CAD build for the part. Positions are in the model's coordinates, mm. A direction names the side the tool comes from. Give positions to 0.01 mm unless a question says otherwise; leave off trailing zeros. Write each loop counter-clockwise with the first axis right and the second up, starting at its lowest first coordinate (ties: lowest second). Pieces come first, ordered by that corner, then holes. Notation, with made-up numbers: (26.5, 36) - (82.5, 36) arc R16 cw to (82.5, 50) - close; hole circle Ø10 at (4, -5.75). An arc over 180 degrees is marked (long way). Answer as a JSON object with one key per item and string values.
from build123d import *

# Parameters (mm, degrees)
F1_DEPTH = 37.5
F2_DEPTH = 20
F4_DEPTH = 70
F3_R     = 5
F5_DEPTH = 30
F6_R     = 20
F7_DEPTH = 100


with BuildPart() as f1:
    # F0 (on Front) → F1 (new body, symmetric)
    with BuildSketch(Plane.XZ):
        with BuildLine():
            ThreePointArc((10.173274, -20.068744), (19.172228, -11.776064), (22.5, 0))
            ThreePointArc((22.5, 0), (19.172228, 11.776064), (10.173274, 20.068744))
            ThreePointArc((10.173274, 20.068744), (-22.5, 0), (10.173274, -20.068744))
        make_face()
    extrude(amount=F1_DEPTH, both=True)

    # F0 (on Front) → F2 (join, symmetric)
    with BuildSketch(Plane.XZ):
        with BuildLine():
            ThreePointArc((10.173274, 20.068744), (19.172228, 11.776064), (22.5, 0))
            ThreePointArc((22.5, 0), (19.172228, -11.776064), (10.173274, -20.068744))
            Line((10.173274, -20.068744), (42.5, -20.285756))
            Line((42.5, -20.285756), (42.5, 0))
            Line((42.5, 0), (42.5, 20.285756))
            Line((42.5, 20.285756), (10.173274, 20.068744))
        make_face()
    extrude(amount=F2_DEPTH, both=True)

    # F3 (on face) → F4 (cut)
    with BuildSketch(Plane(origin=(-0.134258, 0, 19.999549), x_dir=(0.999977, 0, 0.006713), z_dir=(-0.006713, 0, 0.999977))):
        with BuildLine():
            ThreePointArc((40.021521, 5.68982), (41.950542, 3.130714), (42.635219, 0))
            Line((42.635219, 0), (42.635219, 20))
            Line((42.635219, 20), (23.358133, 20))
            Line((23.358133, 20), (40.021521, 5.68982))
        make_face()
        with BuildLine():
            Line((42.635219, -20), (42.635219, 0))
            ThreePointArc((42.635219, 0), (41.950542, -3.130714), (40.021521, -5.68982))
            Line((40.021521, -5.68982), (23.358133, -20))
            Line((23.358133, -20), (42.635219, -20))
        make_face()
    extrude(amount=-F4_DEPTH, mode=Mode.SUBTRACT)

    # F3 (on face) → F5 (cut)
    with BuildSketch(Plane(origin=(-0.134258, 0, 19.999549), x_dir=(0.999977, 0, 0.006713), z_dir=(-0.006713, 0, 0.999977))):
        with Locations((35.135219, 0)):
            Circle(F3_R)
    extrude(amount=-F5_DEPTH, mode=Mode.SUBTRACT)

    # F6 (on face) → F7 (cut)
    with BuildSketch(Plane.XZ.offset(37.5)):
        Circle(F6_R)
    extrude(amount=-F7_DEPTH, mode=Mode.SUBTRACT)


solid = f1.part
Item 1: Cut at C-C (z = 17). State how many separate pieces and enclosed holes the cut face has, and give its area (3 significant figures).
Entries:
{"separate pieces": "2", "enclosed holes": "1", "area": "1,340 mm2"}
Item 2: Probe line 1 (Z direction, x = 0, y = -22); line 2 (X direction, y = 0.5, z = 7.5); line 3 (X direction, y = 23.5, z = -3). List the from-to ranges inside material, lowest first. Write a range as from..to.
Entries:
{"line 1": "-22.5..-20, 20..22.5", "line 2": "-21.21..-18.54, 18.54..30.11, 40.06..42.5", "line 3": "-22.3..-19.77, 19.77..22.3"}
Item 3: Which spindle directions (+Z, -Z, +X, -X, +Y, -Y) get a long thin tool onto all of the face, cutting with end or side? Do faces 1 (the flat face through (23, -20, 2)), 2 (the cylindrical face through (41.6, 3.8, 0.3)), 3 (the flat face through (42.5, 0, -5)), 4 (the flat face through (23, 20, 2)), 5 (the flat face through (-20.1, -37.5, -1.6)). Say none if no direction does.
Entries:
{"face 1": "+X, -Y", "face 2": "+Z, +X, +Y", "face 3": "+Z, -Z, +X, +Y, -Y", "face 4": "+X, +Y", "face 5": "+Z, -Z, +X, -X, -Y"}
Item 4: Mould opens along X. For faces 6 (the cylindrical face through (41.64, -3.73, 0.28)), 7 (the flat face through (-20.1, 37.5, -1.6)), 8 (the cylindrical face through (-4.336, -0.525, -19.524)), 9 (the cylindrical face through (30.104, 0.22, 5.412)) say: +X half, -X half, draft (parallel to the pull), parting line (faces both ways), or undercut.
Entries:
{"face 6": "+X half", "face 7": "draft", "face 8": "undercut", "face 9": "undercut"}
Item 5: Cut at D-D (x = -16.5). Give the cut face in (y, z), and give its area (3 significant figures).
Entries:
{"outline": "(-37.5, -15.3) - (37.5, -15.3) - (37.5, -11.3) - (-37.5, -11.3) - close; (-37.5, 11.3) - (37.5, 11.3) - (37.5, 15.3) - (-37.5, 15.3) - close", "area": "599 mm2"}
Item 6: Flat gauge pins, fed straight in: P1, Ø1, axis at y = -22, z = 9.5, coming from the +X side; P2, Ø12, axis at x = 20.5, y = -28, coming from the -Z side; P3, Ø6, axis at x = 25, z = 9, coming from the -Y side. Where does each tip first touch, or does it go through?
Entries:
{"P1": "x = 20.62", "P2": "z = -17.2", "P3": "y = -20"}
Item 7: Cut at A-A (x = 0). Give the cut face in (y, z).
Entries:
{"outline": "(-37.5, -22.5) - (37.5, -22.5) - (37.5, -20) - (-37.5, -20) - close; (-37.5, 20) - (37.5, 20) - (37.5, 22.5) - (-37.5, 22.5) - close"}
Item 8: Cut at B-B (y = 31). Give the cut face in (x, z).
Entries:
{"outline": "(10.17, -20.07) arc R22.5 ccw to (22.5, 0) arc R22.5 ccw to (10.17, 20.07) arc R22.5 ccw (long way) to start; hole circle Ø40 at (0, 0)"}
